```python
from build123d import *

# Parameters (mm, degrees)
SKETCH1_R               = 38
BOSS_EXTRUDE1_DEPTH     = 10
SKETCH2_W               = 32
SKETCH2_H               = 68.934751758
BOSS_EXTRUDE2_DEPTH     = 38
CUT_EXTRUDE1_DEPTH      = 38
CUT_EXTRUDE1_DEPTH_BACK = 38
SKETCH3_R               = 10
FILLET3_R               = 30
FILLET6_R               = 1


with BuildPart() as part:
    # Sketch1 → Boss-Extrude1 (new body)
    with BuildSketch(Plane(origin=(0, 0, 0), x_dir=(1, 0, 0), z_dir=(0, 1, 0))):
        with Locations(Location((0, 0, 0), (0, 0, 270))):
            Circle(SKETCH1_R)
    extrude(amount=BOSS_EXTRUDE1_DEPTH)

    # Sketch2 → Boss-Extrude2 (add)
    with BuildSketch(Plane(origin=(0, 10, 0), x_dir=(1, 0, 0), z_dir=(0, 1, 0))):
        Rectangle(SKETCH2_W, SKETCH2_H)
    extrude(amount=BOSS_EXTRUDE2_DEPTH)

    # Sketch3 → Cut-Extrude1 (cut, two sides: drawn at the far end of the back side and taken through both)
    with BuildSketch(Plane(origin=(0, 0, 0), x_dir=(0, 0, -1), z_dir=(1, 0, 0)).offset(-CUT_EXTRUDE1_DEPTH_BACK)):
        with Locations(Location((0, 32, 0), (0, 0, 180))):
            Circle(SKETCH3_R)
    extrude(amount=CUT_EXTRUDE1_DEPTH + CUT_EXTRUDE1_DEPTH_BACK, mode=Mode.SUBTRACT)

    # Fillet3
    fillet3_edges = [part.edges().sort_by_distance(p)[0] for p in [
        (0, 48, -34.467375879),
        (0, 48, 34.467375879),
    ]]
    fillet(fillet3_edges, radius=FILLET3_R)

    # Fillet6
    fillet6_edges = [part.edges().sort_by_distance(p)[0] for p in [
        (16, 32, -10),
        (-16, 32, -10),
    ]]
    fillet(fillet6_edges, radius=FILLET6_R)


solid = part.part
```
Work out the finished part from the listing and answer in its coordinate system (mm). A direction names the side the tool comes from. Give positions to 0.01 mm unless a question says otherwise; leave off trailing zeros. Loops run counter-clockwise (first coordinate to the right, second up) from the corner with the lowest first, then second, coordinate; pieces in that order, holes last. Notation, with made-up numbers: M 89.25,39 L 103.25,39 A23 ccw 103.25,67 Z; hole C -37,71 d7. An arc over 180 degrees is marked long. One line per item, written item: value. Start each with the question number.
1. Each of these flat-tipped pins is pushed along its axis until it touches: P1, Ø5, axis at x = 13.5, y = 31, coming from the +Z side; P2, Ø10, axis at y = 34.5, z = 18, coming from the -X side; P3, Ø11, axis at x = 30, z = -15, coming from the +Y side; P4, Ø1, axis at x = -13, z = -29.5, coming from the -Y side. Where does it stop, or does it pass through?
2. Find section C-C (y = 32). Give the vertices of the cut face in (x, z), and give its area (3 significant figures).
3. Find section A-A (z = 0). Give the vertices of the cut face in (x, y).
4. Find the intervals of material crossed by probe 1 along Y at (x, z) = (-3, 0); probe 2 along X at (y, z) = (43.5, -13); probe 3 along Y at (x, z) = (-10, -1), in increasing order.
5. Find section B-B (x = 0). Give the vertices of the cut face in (y, z).
6. Find section D-D (z = 33). Give the vertices of the cut face in (x, y).
7. Determine the mould class of faces 1 (the face through (0.22, 38.98, -25.91)), 2 (the face through (0.22, 38.98, 25.91)), 3 (the face through (-0.21, 41.76, -2.17)) for opening direction Z: released by +Z, released by -Z, zero draft, split by the parting line, or undercut.
8. Which of the six approach directions +Z, -Z, +X, -X, +Y, -Y give full straight-line access (tool end or side, diameter ignored) to faces 4 (the face through (25, 10, 0)), 5 (the face through (-24, 10, 0)), 6 (the face through (0, 10, 36)), 7 (the face through (0, 14, -34.467))?
Reported:
1. P1: stops at z = 32.57
1. P2: stops at x = -16
1. P3: stops at y = 10
1. P4: stops at y = 0
2. outline: M -16,-31 L 16,-31 L 16,-11 A1 ccw 15,-10 L -15,-10 A1 ccw -16,-11 Z; M -16,11 A1 ccw -15,10 L 15,10 A1 ccw 16,11 L 16,31 L -16,31 Z
2. area: 1,340 mm²
3. outline: M -38,0 L 38,0 L 38,10 L 16,10 L 16,21 A1 ccw 15,22 L -15,22 A1 ccw -16,21 L -16,10 L -38,10 Z; M -16,43 A1 ccw -15,42 L 15,42 A1 ccw 16,43 L 16,48 L -16,48 Z
4. probe 1: y = 0 to 22, 42 to 48
4. probe 2: x = -16 to 16
4. probe 3: y = 0 to 22.05, 41.95 to 48
5. outline: M 0,-38 L 10,-38 L 10,-34.47 L 18,-34.47 A30 ccw 48,-4.47 L 48,4.47 A30 ccw 18,34.47 L 10,34.47 L 10,38 L 0,38 Z; hole C 32,0 d20
6. outline: M -18.84,0 L 18.84,0 L 18.84,10 L 16,10 L 16,27.27 L -16,27.27 L -16,10 L -18.84,10 Z
7. face 1: released by -Z
7. face 2: released by +Z
7. face 3: undercut
8. face 4: +Z, -Z, +X, +Y
8. face 5: +Z, -Z, -X, +Y
8. face 6: +Z, +X, -X, +Y
8. face 7: -Z, +X, -X, +Y
